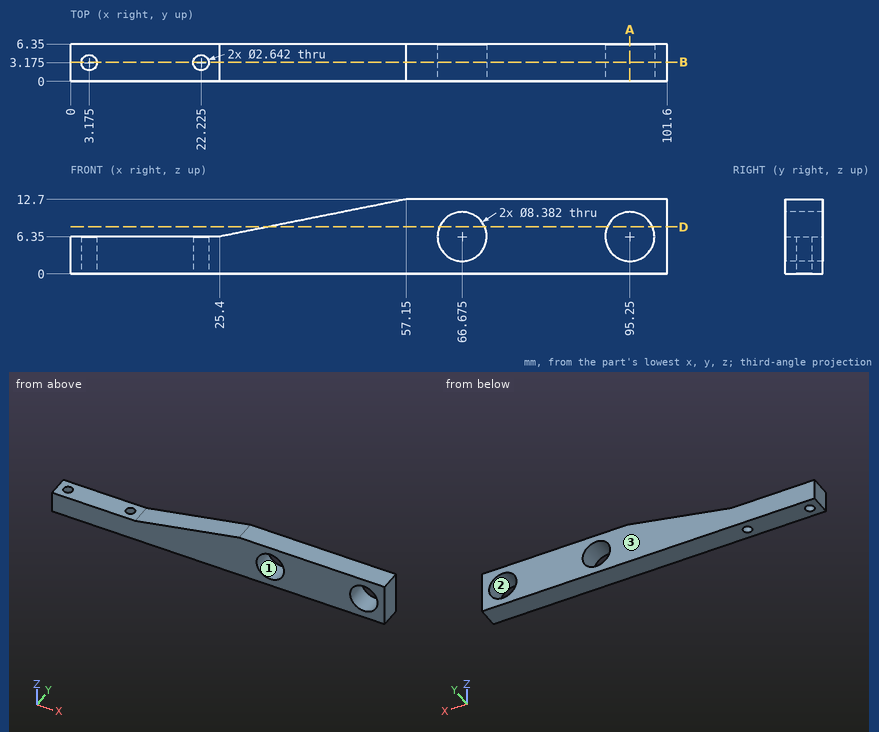
Answer from the drawing. Dimensions are ordinates in mm from the lowest x, y and z of the part. Round coordinates to 2 decimals unless told otherwise and drop trailing zeros. Write each loop counter-clockwise with the first axis right and the second up, starting at its lowest first coordinate (ties: lowest second). Pieces come first, ordered by that corner, then holes. Notation, with made-up numbers: (9.25, -4) -> (14.25, -4) arc R12 ccw to (14.25, 3) -> close; hole circle Ø5 at (40, 67). An arc over 180 degrees is marked (long way). Write each question's results on one line, items separated by ' | '.
1) For a pull along X with two mould halves and no side action, classify the marked faces 1, 2 and 3 as +X half, -X half, draft (parallel to the pull), parting line (faces both ways), or undercut.
Findings:
face 1: undercut | face 2: undercut | face 3: draft
2) The part is cut by section B-B (y = 3.25). State how many separate pieces and enclosed holes the cut face has.
Findings:
separate pieces: 3 | enclosed holes: 2
3) Flat-ended cylindrical pins translate along their axes: pin 1 (3 mm diameter, centred on x = 17, y = 4, fed in from +Z); pin 2 (2 mm diameter, centred on x = 64.5, y = 5, fed in from -Z). Find the tip coordinate at first contact, or state that the pin passes through.
Findings:
pin 1: stops at z = 6.35 | pin 2: stops at z = 0
4) The part is cut by section D-D (z = 8). Write down the section's boundary in (x, y).
Findings:
outline: (33.65, 0) -> (62.82, 0) -> (62.82, 6.35) -> (33.65, 6.35) -> close; (70.53, 0) -> (91.4, 0) -> (91.4, 6.35) -> (70.53, 6.35) -> close; (99.1, 0) -> (101.6, 0) -> (101.6, 6.35) -> (99.1, 6.35) -> close
5) Consider line 1 along Z through (x, y) = (95.25, 3); line 2 along X through (y, z) = (1.5, 6.25) (1 decimal); line 3 along Z through (x, y) = (65.5, 3.75). Determine where each line is inside the solid, lowest interval first. Write a range as [from, to].
Findings:
line 1: z = [0, 2.16], [10.54, 12.7] | line 2: x = [0, 62.5], [70.9, 91.1], [99.4, 101.6] | line 3: z = [0, 2.33], [10.37, 12.7]
6) The part is cut by section A-A (x = 95.25). Write down the section's boundary in (y, z), and give its area (3 significant figures).
Findings:
outline: (0, 0) -> (6.35, 0) -> (6.35, 2.16) -> (0, 2.16) -> close; (0, 10.54) -> (6.35, 10.54) -> (6.35, 12.7) -> (0, 12.7) -> close | area: 27.4 mm²
